Can you work these out from the model? Positions are in its coordinate system, mm. Coordinates: 2 decimals unless noted, no trailing zeros. Order: outer loops, then holes, each group sorted by start corner. A loop starts at its lowest first (then second) coordinate and runs counter-clockwise, first axis right, second up. Notation, with made-up numbers: (-29, 35.5) -> (4, 35.5) arc R31 cw to (4, 62.5) -> close; hole circle Ø4 at (44.5, 11). An arc over 180 degrees is marked (long way). Answer in a Markdown table with one row per item. Add a question column.
1. Imagine slicing it at A-A on y = 0. Write out the boundary of the cut face in (x, z), plus the area to 4 significant figures.
2. Will these pins go through, and if not, where does the flat tip stop? pin 1 (5 mm diameter, centred on x = 79.5, y = -12, fed in from -Z) (1 decimal); pin 2 (6 mm diameter, centred on x = 58.5, z = 3.5, fed in from -Y); pin 3 (5 mm diameter, centred on y = -15, z = 6, fed in from -X); pin 4 (1 mm diameter, centred on y = 46, z = 8, fed in from -X).
3. Imagine slicing it at D-D on x = 67. Write out the boundary of the cut face in (y, z).
4. If I drill on line 1 along Y through (x, z) = (90, 4.25); line 2 along Y through (x, z) = (46.5, 5.5); line 3 along Y through (x, z) = (-33, 4), over which ranges is the centre line in solid material (lowest first)? Write a range as [from, to].
5. Imagine slicing it at C-C on z = 6. Write out the boundary of the cut face in (x, y), plus the area to 3 significant figures.
6. Imagine slicing it at B-B on x = -18.5. Write out the boundary of the cut face in (y, z), plus the area to 3 significant figures.
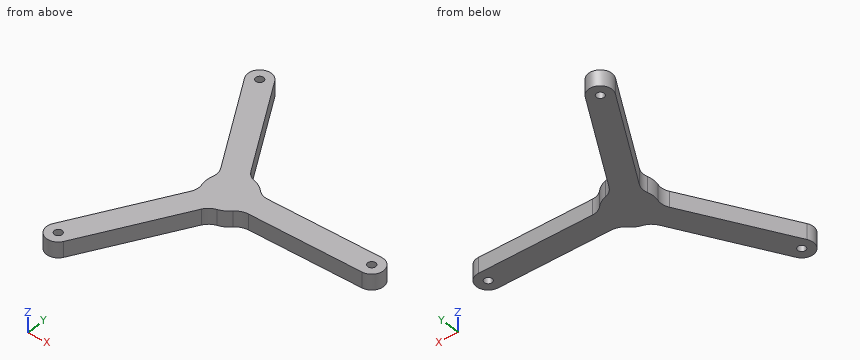
from build123d import *

# Parameters (mm, degrees)
SKETCH1_R                = 2.5
BOSS_EXTRUDE1_DEPTH      = 10
FILLET1_R                = 10
CIRPATTERN2_COUNT        = 3
FILLET1_OF_CIRPATTERN2_R = 10


with BuildPart() as part:
    # Sketch1 → Boss-Extrude1 (new body)
    with BuildSketch(Plane.XY):
        with BuildLine():
            Line((12.990381057, -7.5), (90, -7.5))
            ThreePointArc((90, -7.5), (97.5, 0), (90, 7.5))
            Line((90, 7.5), (12.990381057, 7.5))
            ThreePointArc((12.990381057, 7.5), (-15, 0), (12.990381057, -7.5))
        make_face()
        with Locations((90, 0)):
            Circle(SKETCH1_R, mode=Mode.SUBTRACT)
    boss_extrude1 = extrude(amount=BOSS_EXTRUDE1_DEPTH)

    # Fillet1
    fillet1_edges = [part.edges().sort_by_distance(p)[0] for p in [
        (12.990381057, -7.5, 5),
        (12.990381057, 7.5, 5),
    ]]
    fillet(fillet1_edges, radius=FILLET1_R)

    # CirPattern2: Boss-Extrude1 ×3 about axis
    cirpattern2_axis = Axis((0, 0, 0), (0, 0, 1))
    for i in range(1, CIRPATTERN2_COUNT):
        add(boss_extrude1.rotate(cirpattern2_axis, i * 360 / CIRPATTERN2_COUNT))

    # Fillet1 of CirPattern2
    fillet1_of_cirpattern2_edges = [part.edges().sort_by_distance(p)[0] for p in [
        (0, 15, 5),
        (-12.990381057, 7.5, 5),
        (-12.990381057, -7.5, 5),
        (0, -15, 5),
    ]]
    fillet(fillet1_of_cirpattern2_edges, radius=FILLET1_OF_CIRPATTERN2_R)


solid = part.part
Answers follow:
| question | item | result |
|---|---|---|
| 1 | outline | (-15, 0) -> (87.5, 0) -> (87.5, 10) -> (-15, 10) -> close; (92.5, 0) -> (97.5, 0) -> (97.5, 10) -> (92.5, 10) -> close |
| 1 | area | 1,075 mm² |
| 2 | pin 1 | passes through |
| 2 | pin 2 | stops at y = -7.5 |
| 2 | pin 3 | stops at x = -18.76 |
| 2 | pin 4 | stops at x = -35.51 |
| 3 | outline | (-7.5, 0) -> (7.5, 0) -> (7.5, 10) -> (-7.5, 10) -> close |
| 4 | line 1 | y = [-7.5, -2.5], [2.5, 7.5] |
| 4 | line 2 | y = [-7.5, 7.5] |
| 4 | line 3 | y = [-72.16, -42.16], [42.16, 72.16] |
| 5 | outline | (-51.5, -74.19) arc R7.5 ccw to (-38.5, -81.69) -> (-2.43, -19.21) arc R10 cw to (3.74, -14.53) arc R15 ccw to (10.71, -10.5) arc R10 cw to (17.85, -7.5) -> (90, -7.5) arc R7.5 ccw to (90, 7.5) -> (17.85, 7.5) arc R10 cw to (10.71, 10.5) arc R15 ccw to (3.74, 14.53) arc R10 cw to (-2.43, 19.21) -> (-38.5, 81.69) arc R7.5 ccw to (-51.5, 74.19) -> (-15.42, 11.71) arc R10 cw to (-14.45, 4.03) arc R15 ccw to (-14.45, -4.03) arc R10 cw to (-15.42, -11.71) -> close; hole circle Ø5 at (-45, -77.94); hole circle Ø5 at (-45, 77.94); hole circle Ø5 at (90, 0) |
| 5 | area | 4,330 mm² |
| 6 | outline | (-47.04, 0) -> (-17.04, 0) -> (-17.04, 10) -> (-47.04, 10) -> close; (17.04, 0) -> (47.04, 0) -> (47.04, 10) -> (17.04, 10) -> close |
| 6 | area | 600 mm² |
